Could you check a few things on this model? Use its own coordinates, in mm. A direction names the side the tool comes from. Round coordinates to 2 decimals unless told otherwise and drop trailing zeros. Loops run counter-clockwise (first coordinate to the right, second up) from the corner with the lowest first, then second, coordinate; pieces in that order, holes last.
from build123d import *

# Parameters (mm, degrees)
F0_R     = 60
F0_R_2   = 40
F1_DEPTH = 80
F2_R     = 8.25
F2_R_2   = 60
F3_DEPTH = 25
F5_DEPTH = 80.001


with BuildPart() as f1:
    # F0 (on Front) → F1 (new body)
    with BuildSketch(Plane.XZ):
        Circle(F0_R)
        Circle(F0_R_2, mode=Mode.SUBTRACT)
    extrude(amount=F1_DEPTH)

    # F2 (on face) → F3 (join)
    with BuildSketch(Plane.XZ.offset(80)):
        with BuildLine():
            Line((99.752968, -32.777209), (21.490589, 102.777209))
            ThreePointArc((21.490589, 102.777209), (0, 105), (-21.490589, 102.777209))
            Line((-21.490589, 102.777209), (-99.752968, -32.777209))
            ThreePointArc((-99.752968, -32.777209), (-90.932667, -52.5), (-78.262379, -70))
            Line((-78.262379, -70), (78.262379, -70))
            ThreePointArc((78.262379, -70), (90.932667, -52.5), (99.752968, -32.777209))
        make_face()
        with Locations((-80.540363, -46.5)):
            Circle(F2_R, mode=Mode.SUBTRACT)
        with Locations((80.540363, -46.5)):
            Circle(F2_R, mode=Mode.SUBTRACT)
        Circle(F2_R_2, mode=Mode.SUBTRACT)
        with Locations((0, 93)):
            Circle(F2_R, mode=Mode.SUBTRACT)
    extrude(amount=-F3_DEPTH)

    # F4 (on face) → F5 (cut, through all)
    with BuildSketch(Plane.XZ.offset(80)):
        with BuildLine():
            Line((11, 45.4), (-11, 45.4))
            Line((-11, 45.4), (-11, 38.457769))
            ThreePointArc((-11, 38.457769), (0, 40), (11, 38.457769))
            Line((11, 38.457769), (11, 45.4))
        make_face()
    extrude(amount=-F5_DEPTH, mode=Mode.SUBTRACT)


solid = f1.part
Item 1: If I drill on line 1 along Z through (x, y) = (0, -71); line 2 along Y through (x, z) = (-41.5, -60.5); line 3 along Z through (x, y) = (-4, -22), over which ranges is the centre line in solid material (lowest first)?
Results list:
line 1: z = -70 to -40, 45.4 to 84.75, 101.25 to 105
line 2: y = -80 to -55
line 3: z = -59.87 to -39.8, 45.4 to 59.87
Item 2: Will these pins go through, and if not, where does the flat tip stop? pin 1 (15 mm diameter, centred on x = 80.54, z = -46.5, fed in from -Y); pin 2 (8 mm diameter, centred on x = 42.5, y = -44, fed in from -Z); pin 3 (6 mm diameter, centred on x = -32, y = -59, fed in from +Z); pin 4 (10 mm diameter, centred on y = -61.5, z = 61, fed in from +X).
Results list:
pin 1: passes through
pin 2: stops at z = -46.02
pin 3: stops at z = 89.77
pin 4: stops at x = 48.5
Item 3: We'd pull the mould along X, two halves only. Please class faces 1 (the flat face through (61.17, -67.68, 34.05)), 2 (the flat face through (-11, -41, 42)), 3 (the cylindrical face through (-91.08, -67.68, -52.24)): released by +X, released by -X, zero draft, split by the parting line, or undercut.
Results list:
face 1: released by +X
face 2: undercut
face 3: released by -X
Item 4: If we section it at B-B, the plane x = 0: Please give me the cut outline in (y, z), then the cut area to 3 significant figures.
Results list:
outline: (-80, -70) - (-55, -70) - (-55, -60) - (0, -60) - (0, -40) - (-80, -40) - close; (-80, 45.4) - (0, 45.4) - (0, 60) - (-55, 60) - (-55, 84.75) - (-80, 84.75) - close; (-80, 101.25) - (-55, 101.25) - (-55, 105) - (-80, 105) - close
area: 3,730 mm2
Item 5: For faces 4 (the flat face through (11, -41, 42)), 5 (the flat face through (7, -55, -60)), 6 (the flat face through (-1, -68, -70)), which set-ups out of +Z, -Z, +X, -X, +Y, -Y let a thin tool reach every point of the face, with its end or its side?
Results list:
face 4: +Y, -Y
face 5: +Y
face 6: -Z, +X, -X, +Y, -Y
Item 6: If we section it at D-D, the plane z = -46.5: Please give me the cut outline in (x, y), then the cut area to 3 significant figures.
Results list:
outline: (-94.14, -80) - (-88.79, -80) - (-88.79, -55) - (-94.14, -55) - close; (-72.29, -80) - (72.29, -80) - (72.29, -55) - (37.92, -55) - (37.92, 0) - (-37.92, 0) - (-37.92, -55) - (-72.29, -55) - close; (88.79, -80) - (94.14, -80) - (94.14, -55) - (88.79, -55) - close
area: 8,050 mm2
Item 7: If we section it at C-C, the plane z = 93: Please give me the cut outline in (x, y).
Results list:
outline: (-27.14, -80) - (-8.25, -80) - (-8.25, -55) - (-27.14, -55) - close; (8.25, -80) - (27.14, -80) - (27.14, -55) - (8.25, -55) - close
Item 8: If we section it at A-A, the plane y = -61.5: Please give me the cut outline in (x, z), then the cut area to 3 significant figures.
Results list:
outline: (-99.75, -32.78) arc R105 ccw to (-78.26, -70) - (78.26, -70) arc R105 ccw to (99.75, -32.78) - (21.49, 102.78) arc R105 ccw to (-21.49, 102.78) - close; hole circle Ø16.5 at (-80.54, -46.5); hole (-11, 38.46) arc R40 ccw (long way) to (11, 38.46) - (11, 45.4) - (-11, 45.4) - close; hole circle Ø16.5 at (0, 93); hole circle Ø16.5 at (80.54, -46.5)
area: 17,500 mm2
